from build123d import *

# Parameters (mm, degrees)
BOSS_EXTRUDE1_DEPTH      = 9
BOSS_EXTRUDE1_DEPTH_BACK = 9
SKETCH1_R                = 5
CUT_EXTRUDE1_DEPTH       = 12.445523142
CUT_EXTRUDE1_DEPTH_BACK  = 12.445523142
SKETCH7_R                = 2.5
SKETCH8_W                = 10.865587176
SKETCH8_H                = 1
CUT_EXTRUDE2_DEPTH       = 2


with BuildPart() as part:
    # Sketch1 → Boss-Extrude1 (new, two sides: drawn at the far end of the back side and taken through both)
    with BuildSketch(Plane(origin=(0, 0, 0), x_dir=(0, 0, -1), z_dir=(1, 0, 0)).offset(-BOSS_EXTRUDE1_DEPTH_BACK)):
        Circle(SKETCH1_R)
    extrude(amount=BOSS_EXTRUDE1_DEPTH + BOSS_EXTRUDE1_DEPTH_BACK)

    # Sketch7 → Cut-Extrude1 (cut, two sides: drawn at the far end of the back side and taken through both)
    with BuildSketch(Plane(origin=(0, 0, 0), x_dir=(1, 0, 0), z_dir=(0, 1, 0)).offset(-CUT_EXTRUDE1_DEPTH_BACK)):
        with Locations(Location((0, 0, 0), (0, 0, 270))):
            Circle(SKETCH7_R)
    extrude(amount=CUT_EXTRUDE1_DEPTH + CUT_EXTRUDE1_DEPTH_BACK, mode=Mode.SUBTRACT)

    # Sketch8 → Cut-Extrude2 (cut)
    with BuildSketch(Plane(origin=(9, 0, 0), x_dir=(0, 0, -1), z_dir=(1, 0, 0))):
        Rectangle(SKETCH8_W, SKETCH8_H)
    extrude(amount=-CUT_EXTRUDE2_DEPTH, mode=Mode.SUBTRACT)


solid = part.part
Build history of the part. All positions in model axes, mm. A direction names the side the tool comes from. Give positions to 0.01 mm unless a question says otherwise; leave off trailing zeros. Write each loop counter-clockwise with the first axis right and the second up, starting at its lowest first coordinate (ties: lowest second). Pieces come first, ordered by that corner, then holes. Notation, with made-up numbers: (-25.75, 13) - (17.25, 13) arc R18 cw to (17.25, 19) - close; hole circle Ø3 at (24.25, -22.5). An arc over 180 degrees is marked (long way). Use one line per item in the form item = value. Start each with the question number.
1. Probe line 1 (X direction, y = 0, z = 0); line 2 (X direction, y = -1.5, z = 0); line 3 (Y direction, x = 8.25, z = 0). List the from-to ranges inside material, lowest first. Write a range as [from, to].
2. Band-saw the part on D-D on z = 2. Write the cut outline in (x, y).
3. Two-plate mould, pull along X, no slides. Class faces 1 (the face through (-9, 0, 0)), 2 (the face through (7, 0, 0)), 3 (the face through (0.751, -0.07, 2.385)), 4 (the face through (8, -0.5, 0)): released by +X, released by -X, zero draft, split by the parting line, or undercut.
4. 3-axis set-ups, long thin cutter, end or side, ignore diameter. For faces 5 (the face through (9, 2, 0)), 6 (the face through (8, 0.5, 0)): which of +Z, -Z, +X, -X, +Y, -Y reach the whole face in a straight line?
5. Band-saw the part on C-C on x = 0. Write the cut outline in (y, z).
6. Band-saw the part on B-B on y = 0. Write the cut outline in (x, z), plus the area to 3 significant figures.
7. Drop flat-ended pins along their axis: pin 1 Ø5 at (x, z) = (3, 3.5) entering from +Y; pin 2 Ø4 at (x, z) = (6, -3.5) entering from +Y; pin 3 Ø0.8 at (y, z) = (0, -1) entering from +X. Give the stop position or say it passes through.
8. Band-saw the part on A-A on z = 0. Write the cut outline in (x, y).
Conclusion:
q1.line_1 = [-9, -2.5], [2.5, 7]
q1.line_2 = [-9, -2.5], [2.5, 9]
q1.line_3 = [-5, -0.5], [0.5, 5]
q2.outline = (-9, -4.58) - (-1.5, -4.58) - (-1.5, 4.58) - (-9, 4.58) - close; (1.5, -4.58) - (9, -4.58) - (9, -0.5) - (7, -0.5) - (7, 0.5) - (9, 0.5) - (9, 4.58) - (1.5, 4.58) - close
q3.face_1 = released by -X
q3.face_2 = released by +X
q3.face_3 = undercut
q3.face_4 = zero draft
q4.face_5 = +Z, -Z, +X, +Y, -Y
q4.face_6 = +Z, -Z, +X
q5.outline = (-4.33, -2.5) arc R5 ccw to (4.33, -2.5) - close; (-4.33, 2.5) - (4.33, 2.5) arc R5 ccw to start
q6.outline = (-9, -5) - (7, -5) - (7, 5) - (-9, 5) - close; hole circle Ø5 at (0, 0)
q6.area = 140 mm²
q7.pin_1 = 4.9
q7.pin_2 = 4.77
q7.pin_3 = 7
q8.outline = (-9, -5) - (-2.5, -5) - (-2.5, 5) - (-9, 5) - close; (2.5, -5) - (9, -5) - (9, -0.5) - (7, -0.5) - (7, 0.5) - (9, 0.5) - (9, 5) - (2.5, 5) - close
